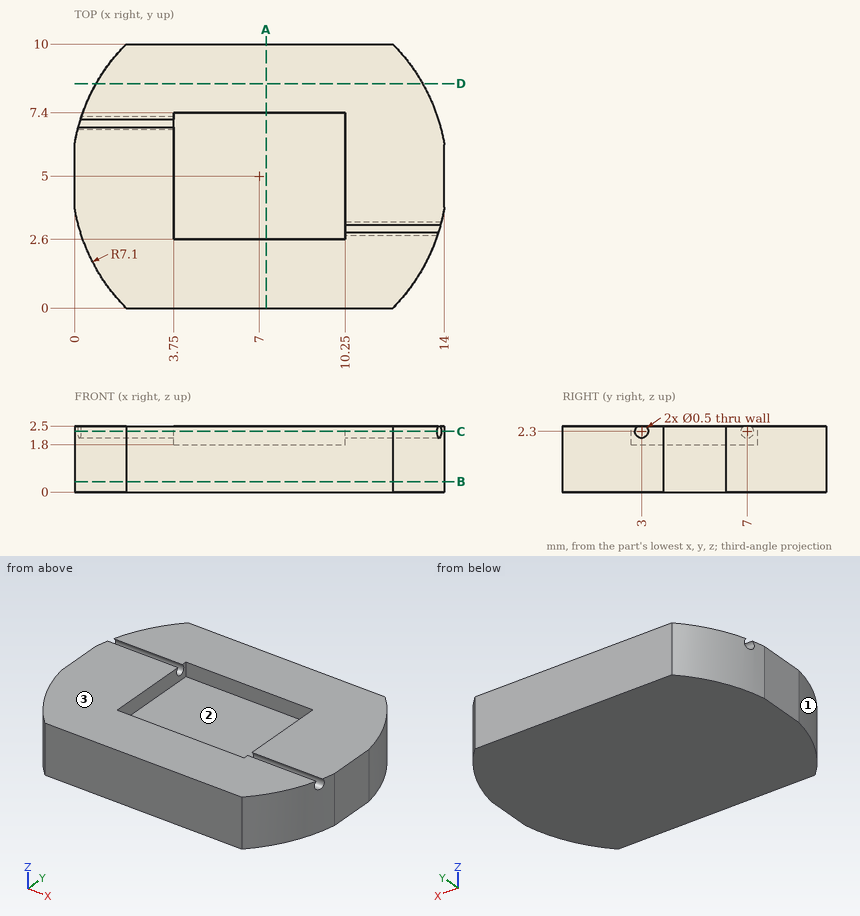
For this review, use the dimensioned drawing (mm, ordinates from the lowest corner) and the shaded views. Coordinates: 2 decimals unless noted, no trailing zeros. Order: outer loops, then holes, each group sorted by start corner. A loop starts at its lowest first (then second) coordinate and runs counter-clockwise, first axis right, second up. Notation, with made-up numbers: (83, -35) -> (138, -35) arc R28 cw to (138, -11) -> close; hole circle Ø10 at (-25, 28.25). An arc over 180 degrees is marked (long way). One line per item, written item: value. Start each with the question number.
Q1. Take a section at A-A, the plane x = 7.25. State the section outline as (y, z) points.
Q2. Take a section at B-B, the plane z = 0.4. State the section outline as (x, y) points.
Q3. Insertion check: pin 1 Ø1.5 at (y, z) = (7.5, 0.5) entering from -X; pin 2 Ø1.4 at (x, y) = (7, 5.5) entering from +Z. Each pin has a flat end and moves straight along its axis. Give the tip position at first contact, or say it passes through.
Q4. Take a section at D-D, the plane y = 8.5. State the section outline as (x, z) points.
Q5. Mouldability with a two-part tool opening along X and no side actions: class the marked faces 1, 2 and 3 as pulls with the +X half, pulls with the -X half, needs draft (parallel to the pull), parting line crosses it, or undercut.
Q6. For probe 1 along Y at (x, z) = (11.85, 2.3); probe 2 along Z at (x, y) = (5.5, 3); probe 3 along X at (y, z) = (3.25, 2.1), list the stretches that pass through material, from the lowest coordinate up.
Q7. Take a section at C-C, the plane z = 2.3. State the section outline as (x, y) points, then the cut area to 3 significant figures.
Values follow:
1. outline: (0, 0) -> (10, 0) -> (10, 2.5) -> (7.4, 2.5) -> (7.4, 1.8) -> (2.6, 1.8) -> (2.6, 2.5) -> (0, 2.5) -> close
2. outline: (0, 3.81) arc R7.1 ccw to (1.96, 0) -> (12.04, 0) arc R7.1 ccw to (14, 3.81) -> (14, 6.19) arc R7.1 ccw to (12.04, 10) -> (1.96, 10) arc R7.1 ccw to (0, 6.19) -> close
3. pin 1: stops at x = 0.12
3. pin 2: stops at z = 1.8
4. outline: (0.82, 0) -> (13.18, 0) -> (13.18, 2.5) -> (0.82, 2.5) -> close
5. face 1: pulls with the -X half
5. face 2: undercut
5. face 3: needs draft
6. probe 1: y = 0 to 2.75, 3.25 to 10
6. probe 2: z = 0 to 1.8
6. probe 3: x = 0.12 to 3.75, 10.25 to 13.88
7. outline: (0, 3.81) arc R7.1 ccw to (1.96, 0) -> (12.04, 0) arc R7.1 ccw to (13.73, 2.75) -> (10.25, 2.75) -> (10.25, 2.6) -> (3.75, 2.6) -> (3.75, 6.75) -> (0.12, 6.75) arc R7.1 ccw to (0, 6.19) -> close; (0.27, 7.25) -> (3.75, 7.25) -> (3.75, 7.4) -> (10.25, 7.4) -> (10.25, 3.25) -> (13.88, 3.25) arc R7.1 ccw to (14, 3.81) -> (14, 6.19) arc R7.1 ccw to (12.04, 10) -> (1.96, 10) arc R7.1 ccw to start
7. area: 94.1 mm2
